from build123d import *

# Parameters (mm, degrees)
SKETCH_1_W          = 29
SKETCH_1_H          = 41
EXTRUDE_1_DEPTH     = 47
SKETCH_2_W          = 26.5
SKETCH_2_H          = 38.5
CUT_EXTRUDE_1_DEPTH = 46
SKETCH_4_W          = 6
SKETCH_4_H          = 8
EXTRUDE_2_DEPTH     = 2
SKETCH_5_R          = 1
CUT_EXTRUDE_4_DEPTH = 2


with BuildPart() as part:
    # ｽｹｯﾁ1 → ﾎﾞｽ - 押し出し1 (new body)
    with BuildSketch(Plane.XY):
        Rectangle(SKETCH_1_W, SKETCH_1_H)
    extrude(amount=EXTRUDE_1_DEPTH)

    # ｽｹｯﾁ2 → ｶｯﾄ - 押し出し1 (cut)
    with BuildSketch(Plane.XY):
        Rectangle(SKETCH_2_W, SKETCH_2_H)
    extrude(amount=CUT_EXTRUDE_1_DEPTH, mode=Mode.SUBTRACT)

    # ｽｹｯﾁ4 → ﾎﾞｽ - 押し出し2 (add)
    with BuildSketch(Plane.XY):
        with Locations((17.5, 16.5)):
            Rectangle(SKETCH_4_W, SKETCH_4_H)
        with Locations((17.5, -16.5)):
            Rectangle(SKETCH_4_W, SKETCH_4_H)
        with Locations((-17.5, -16.5)):
            Rectangle(SKETCH_4_W, SKETCH_4_H)
        with Locations((-17.5, 16.5)):
            Rectangle(SKETCH_4_W, SKETCH_4_H)
    extrude(amount=EXTRUDE_2_DEPTH)

    # ｽｹｯﾁ5 → ｶｯﾄ - 押し出し4 (cut)
    with BuildSketch(Plane.XY):
        with Locations((-16, 16)):
            Circle(SKETCH_5_R)
        with Locations((-16, -16)):
            Circle(SKETCH_5_R)
        with Locations((16, -16)):
            Circle(SKETCH_5_R)
        with Locations((16, 16)):
            Circle(SKETCH_5_R)
    extrude(amount=CUT_EXTRUDE_4_DEPTH, mode=Mode.SUBTRACT)


solid = part.part
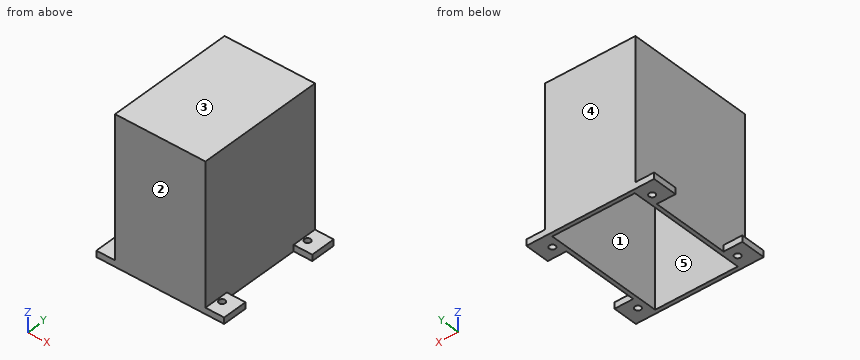
Can you work these out from the model? Positions are in its coordinate system, mm. Face numbers are marked on the shaded views. A direction names the side the tool comes from. Coordinates: 2 decimals unless noted, no trailing zeros. Write each loop counter-clockwise with the first axis right and the second up, starting at its lowest first coordinate (ties: lowest second). Pieces come first, ordered by that corner, then holes. Notation, with made-up numbers: (77.25, 1) -> (134.25, 1) arc R17 cw to (134.25, 25) -> close; hole circle Ø10 at (66, 23). An arc over 180 degrees is marked (long way). Answer as CSV lines item,"result".
1) If we section it at A-A on y = 16: Please give me the cut outline in (x, z), then the cut area to 3 significant figures.
Check result:
outline,"(-20.5, 0) -> (-17, 0) -> (-17, 2) -> (-20.5, 2) -> close; (-15, 0) -> (-13.25, 0) -> (-13.25, 46) -> (13.25, 46) -> (13.25, 0) -> (15, 0) -> (15, 2) -> (14.5, 2) -> (14.5, 47) -> (-14.5, 47) -> (-14.5, 2) -> (-15, 2) -> close; (17, 0) -> (20.5, 0) -> (20.5, 2) -> (17, 2) -> close"
area,"160 mm²"
2) On a 3-axis mill with a long thin cutter (end or side, diameter ignored), from which of +Z, -Z, +X, -X, +Y, -Y can I reach the whole of each face in a straight line? I mean the marked faces 1 and 2. Say none if no direction works.
Check result:
face 1,"-Z"
face 2,"+Z, -Z, +X, -X, -Y"
3) If we section it at C-C on x = 0: Please give me the cut outline in (y, z).
Check result:
outline,"(-20.5, 0) -> (-19.25, 0) -> (-19.25, 46) -> (19.25, 46) -> (19.25, 0) -> (20.5, 0) -> (20.5, 47) -> (-20.5, 47) -> close"
4) If we section it at D-D on x = 16: Please give me the cut outline in (y, z).
Check result:
outline,"(-20.5, 0) -> (-17, 0) -> (-17, 2) -> (-20.5, 2) -> close; (-15, 0) -> (-12.5, 0) -> (-12.5, 2) -> (-15, 2) -> close; (12.5, 0) -> (15, 0) -> (15, 2) -> (12.5, 2) -> close; (17, 0) -> (20.5, 0) -> (20.5, 2) -> (17, 2) -> close"
5) If we mould it in two halves opening along Y, with no side actions, what happens to the marked faces 3, 4 and 5? For each: +Y half, -Y half, draft (parallel to the pull), parting line (faces both ways), or undercut.
Check result:
face 3,"draft"
face 4,"+Y half"
face 5,"undercut"
6) Will these pins go through, and if not, where does the flat tip stop? P1, Ø12, axis at y = -7.5, z = 7.5, coming from the -X side; P2, Ø3, axis at y = 6.5, z = 12, coming from the +X side; P3, Ø3, axis at x = 18, y = 16, coming from the +Z side.
Check result:
P1,"x = -14.5"
P2,"x = 14.5"
P3,"z = 2"
7) If I drill on line 1 (Y direction, x = -16, z = 1.2); line 2 (X direction, y = 2, z = 32.5); line 3 (Y direction, x = 7.5, z = 33), over which ranges is the centre line in solid material (lowest first)? Write a range as from..to.
Check result:
line 1,"-20.5..-17, -15..-12.5, 12.5..15, 17..20.5"
line 2,"-14.5..-13.25, 13.25..14.5"
line 3,"-20.5..-19.25, 19.25..20.5"
8) If we section it at B-B on z = 39.5: Please give me the cut outline in (x, y).
Check result:
outline,"(-14.5, -20.5) -> (14.5, -20.5) -> (14.5, 20.5) -> (-14.5, 20.5) -> close; hole (-13.25, -19.25) -> (13.25, -19.25) -> (13.25, 19.25) -> (-13.25, 19.25) -> close"
